from build123d import *

# Parameters (mm, degrees)
F0_R     = 1
F0_W     = 52
F0_H     = 52
F0_W_2   = 50
F0_H_2   = 50
F1_DEPTH = 2.5
F2_DEPTH = 0.5
F3_W     = 52
F3_H     = 5
F4_DEPTH = 0.5


with BuildPart() as f1:
    # F0 (on Top) → F1 (new body)
    with BuildSketch(Plane.XY):
        with BuildLine():
            Line((57, 0), (5, 0))
            ThreePointArc((5, 0), (1.464466, -1.464466), (0, -5))
            Line((0, -5), (0, -57))
            ThreePointArc((0, -57), (1.464466, -60.535534), (5, -62))
            Line((5, -62), (57, -62))
            ThreePointArc((57, -62), (60.535534, -60.535534), (62, -57))
            Line((62, -57), (62, -5))
            ThreePointArc((62, -5), (60.535534, -1.464466), (57, 0))
        make_face()
        with Locations((3, -59)):
            Circle(F0_R, mode=Mode.SUBTRACT)
        with Locations((59, -59)):
            Circle(F0_R, mode=Mode.SUBTRACT)
        with Locations((3, -3)):
            Circle(F0_R, mode=Mode.SUBTRACT)
        with Locations((31, -31)):
            Rectangle(F0_W, F0_H, mode=Mode.SUBTRACT)
        with Locations((59, -3)):
            Circle(F0_R, mode=Mode.SUBTRACT)
        with Locations((31, -31)):
            Rectangle(F0_W, F0_H)
        with Locations((31, -31)):
            Rectangle(F0_W_2, F0_H_2, mode=Mode.SUBTRACT)
    extrude(amount=F1_DEPTH)

    # F0 (on Top) → F2 (cut)
    with BuildSketch(Plane.XY):
        with Locations((31, -31)):
            Rectangle(F0_W, F0_H)
        with Locations((31, -31)):
            Rectangle(F0_W_2, F0_H_2, mode=Mode.SUBTRACT)
    extrude(amount=F2_DEPTH, mode=Mode.SUBTRACT)

    # F3 (on face) → F4 (cut)
    with BuildSketch(Plane.XY):
        with Locations((31, -2.5)):
            Rectangle(F3_W, F3_H)
    extrude(amount=F4_DEPTH, mode=Mode.SUBTRACT)


solid = f1.part
The model under review builds one solid part; all positions refer to its coordinate system, in mm. A direction names the side the tool comes from. Give positions to 0.01 mm unless a question says otherwise; leave off trailing zeros. Write each loop counter-clockwise with the first axis right and the second up, starting at its lowest first coordinate (ties: lowest second). Pieces come first, ordered by that corner, then holes.
1. Draft analysis for pull direction X (two halves, no side actions). For faces 3 (the flat face through (62, -31, 1)), 4 (the flat face through (25, -5, 0.5)), 5 (the flat face through (5.6, -33.2, 2.5)), state which applies: +X half, -X half, draft (parallel to the pull), parting line (faces both ways), or undercut.
2. Add section B-B, the plane x = 19.5. Write out the cut boundary in (y, z).
3. Wall thickness on L1, parallel to X at y = -28, z = 0.4; L2, parallel to Y at x = 16.5, z = 0.6; L3, parallel to Y at x = 59, z = 0.65: over which ranges is each line inside the solid? List them lowest first.
4. Add section D-D, the plane y = -3. Write out the cut boundary in (x, z), plus the area to 3 significant figures.
5. Tool access review of faces 1 (the cylindrical face through (60, -61, 1)), 2 (the flat face through (56, -31, 1)): name each direction out of +Z, -Z, +X, -X, +Y, -Y from which nothing blocks a thin tool from reaching the whole face with its end or side.
6. Add section A-A, the plane y = -23.5. Write out the cut boundary in (x, z), plus the area to 3 significant figures.
7. Add section C-C, the plane z = 1.55. Write out the cut boundary in (x, y), plus the area to 3 significant figures.
Worked answers:
1. face 3: +X half
1. face 4: undercut
1. face 5: draft
2. outline: (-62, 0) - (-57, 0) - (-57, 0.5) - (-56, 0.5) - (-56, 2.5) - (-62, 2.5) - close; (-6, 0.5) - (0, 0.5) - (0, 2.5) - (-6, 2.5) - close
3. L1: x = 0 to 5, 57 to 62
3. L2: y = -62 to -56, -6 to 0
3. L3: y = -61.58 to -60, -58 to -4, -2 to -0.42
4. outline: (0.42, 0) - (2, 0) - (2, 2.5) - (0.42, 2.5) - close; (4, 0) - (5, 0) - (5, 0.5) - (57, 0.5) - (57, 0) - (58, 0) - (58, 2.5) - (4, 2.5) - close; (60, 0) - (61.58, 0) - (61.58, 2.5) - (60, 2.5) - close
4. area: 117 mm2
5. face 1: +Z, -Z, +X, -Y
5. face 2: +Z, -Z
6. outline: (0, 0) - (5, 0) - (5, 0.5) - (6, 0.5) - (6, 2.5) - (0, 2.5) - close; (56, 0.5) - (57, 0.5) - (57, 0) - (62, 0) - (62, 2.5) - (56, 2.5) - close
6. area: 29.0 mm2
7. outline: (0, -57) arc R5 ccw to (5, -62) - (57, -62) arc R5 ccw to (62, -57) - (62, -5) arc R5 ccw to (57, 0) - (5, 0) arc R5 ccw to (0, -5) - close; hole circle Ø2 at (3, -59); hole circle Ø2 at (3, -3); hole (6, -56) - (56, -56) - (56, -6) - (6, -6) - close; hole circle Ø2 at (59, -59); hole circle Ø2 at (59, -3)
7. area: 1,310 mm2
